```python
from build123d import *

# Parameters (mm, degrees)
BOSS_EXTRUDE1_DEPTH = 25.4
SKETCH3_R           = 6.35
CUT_EXTRUDE1_DEPTH  = 48.941448664
SKETCH2_R           = 2.4892
CUT_EXTRUDE2_DEPTH  = 48.941448664


with BuildPart() as part:
    # Sketch1 → Boss-Extrude1 (new body)
    with BuildSketch(Plane.XY):
        Polygon((0, 0), (0, 25.4), (3.175, 25.4), (3.175, 3.175), (31.75, 3.175), (31.75, 0), align=None)
    extrude(amount=BOSS_EXTRUDE1_DEPTH)

    # Sketch3 → Cut-Extrude1 (cut, through all)
    with BuildSketch(Plane.ZY):
        with Locations((12.7, 12.7)):
            Circle(SKETCH3_R)
    extrude(amount=-CUT_EXTRUDE1_DEPTH, mode=Mode.SUBTRACT)

    # Sketch2 → Cut-Extrude2 (cut, through all)
    with BuildSketch(Plane.XZ):
        with Locations((12.7, 12.7)):
            Circle(SKETCH2_R)
        with Locations((25.4, 12.7)):
            Circle(SKETCH2_R)
    extrude(amount=-CUT_EXTRUDE2_DEPTH, mode=Mode.SUBTRACT)


solid = part.part
```
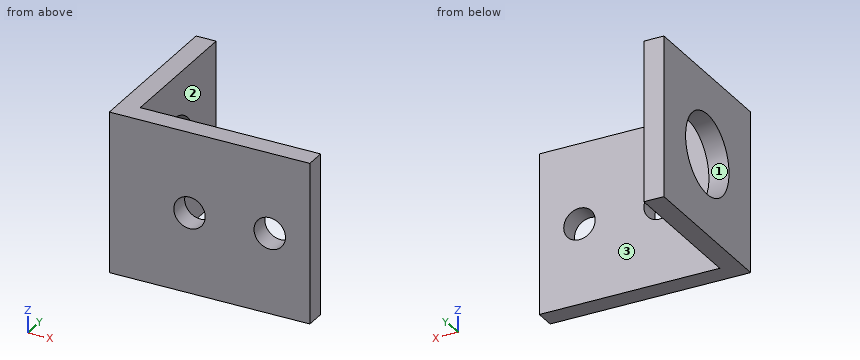
Build history of the part. All positions in model axes, mm. Face numbers are marked on the shaded views. Coordinates: 2 decimals unless noted, no trailing zeros. Order: outer loops, then holes, each group sorted by start corner. A loop starts at its lowest first (then second) coordinate and runs counter-clockwise, first axis right, second up. Notation, with made-up numbers: M 6,63 L 11,63 A17 ccw 11,84 Z; hole C -18,67.25 d2. An arc over 180 degrees is marked long. One line per question, with ' | ' between items. Start each with the question number.
1. Cut at B-B (y = 12.7). Write the cut outline in (x, z) (3 decimals), plus the area to 3 significant figures.
2. Cut at D-D (z = 9.75). Write the cut outline in (x, y) (3 decimals), plus the area to 3 significant figures.
3. Cut at A-A (x = 25.4). Write the cut outline in (y, z) (3 decimals), plus the area to 3 significant figures.
4. Mould opens along Y. For the marked faces 1, 2 and 3 say: +Y half, -Y half, draft (parallel to the pull), parting line (faces both ways), or undercut.
5. Wall check: line 1 along Z through (x, y) = (12.7, 1.6); line 2 along Y through (x, z) = (2.2, 12.7); line 3 along Y through (x, z) = (5.5, 12.5) (3 decimals). Give the ranges that are in metal, low to high. Write a range as [from, to].
6. Flat gauge pins, fed straight in: P1, Ø2, axis at x = 11.5, y = 4.5, coming from the -Z side (3 decimals); P2, Ø7.5, axis at x = 14.5, z = 11, coming from the +Y side (3 decimals); P3, Ø6.5, axis at y = 16, z = 12, coming from the +X side (3 decimals). Where does each tip first touch, or does it go through?
7. Cut at C-C (z = 12.7). Write the cut outline in (x, y) (3 decimals), plus the area to 3 significant figures.
The answers:
1) outline: M 0,0 L 3.175,0 L 3.175,6.35 L 0,6.35 Z; M 0,19.05 L 3.175,19.05 L 3.175,25.4 L 0,25.4 Z | area: 40.3 mm2
2) outline: M 0,0 L 31.75,0 L 31.75,3.175 L 3.175,3.175 L 3.175,7.077 L 0,7.077 Z; M 0,18.323 L 3.175,18.323 L 3.175,25.4 L 0,25.4 Z | area: 136 mm2
3) outline: M 0,0 L 3.175,0 L 3.175,10.211 L 0,10.211 Z; M 0,15.189 L 3.175,15.189 L 3.175,25.4 L 0,25.4 Z | area: 64.8 mm2
4) face 1: undercut | face 2: draft | face 3: +Y half
5) line 1: z = [0, 10.21], [15.19, 25.4] | line 2: y = [0, 6.35], [19.05, 25.4] | line 3: y = [0, 3.175]
6) P1: passes through | P2: stops at y = 3.175 | P3: stops at x = 3.175
7) outline: M 0,0 L 10.211,0 L 10.211,3.175 L 3.175,3.175 L 3.175,6.35 L 0,6.35 Z; M 0,19.05 L 3.175,19.05 L 3.175,25.4 L 0,25.4 Z; M 15.189,0 L 22.911,0 L 22.911,3.175 L 15.189,3.175 Z; M 27.889,0 L 31.75,0 L 31.75,3.175 L 27.889,3.175 Z | area: 99.4 mm2
